Design review of the part built by this model. Coordinates are the model's own, in mm. A direction names the side the tool comes from. Give positions to 0.01 mm unless a question says otherwise; leave off trailing zeros. Loops run counter-clockwise (first coordinate to the right, second up) from the corner with the lowest first, then second, coordinate; pieces in that order, holes last. Notation, with made-up numbers: M 16,22.25 L 61,22.25 A18 cw 61,45.25 Z; hole C 2.5,82.5 d5. An arc over 180 degrees is marked long. Answer as CSV lines item,"result".
```python
from build123d import *

# Parameters (mm, degrees)
BOSS_EXTRUDE1_DEPTH = 36
SKETCH2_W           = 16.184746641
SKETCH2_H           = 32
CUT_EXTRUDE1_DEPTH  = 36
CUT_EXTRUDE2_DEPTH  = 36
SKETCH4_3_R         = 12
CUT_EXTRUDE3_DEPTH  = 36
BOSS_EXTRUDE2_START = 14
SKETCH4_4_R         = 18
SKETCH4_4_R_2       = 12
BOSS_EXTRUDE2_DEPTH = 14
SKETCH5_R           = 4
CUT_EXTRUDE4_DEPTH  = 14
FILLET2_R           = 8
SKETCH9_W           = 12
SKETCH9_H           = 4
BOSS_EXTRUDE3_DEPTH = 12
CUT_EXTRUDE5_DEPTH  = 53


with BuildPart() as part:
    # Sketch1 → Boss-Extrude1 (new body)
    with BuildSketch(Plane(origin=(0, 0, 0), x_dir=(1, 0, 0), z_dir=(0, 1, 0))):
        Polygon((0, 0), (66, 0), (66, 6), (6, 6), (6, 46), (-14, 46), (-14, 14), (0, 14), align=None)
    extrude(amount=BOSS_EXTRUDE1_DEPTH)

    # Sketch2 → Cut-Extrude1 (cut)
    with BuildSketch(Plane(origin=(0, 36, 0), x_dir=(1, 0, 0), z_dir=(0, 1, 0))):
        with Locations((-8.092373321, 30)):
            Rectangle(SKETCH2_W, SKETCH2_H)
    extrude(amount=-CUT_EXTRUDE1_DEPTH, mode=Mode.SUBTRACT)

    # Sketch4 → Cut-Extrude2 (cut)
    with BuildSketch(Plane.ZY):
        with BuildLine():
            ThreePointArc((-23, 0), (-41, 18), (-23, 36))
            Line((-23, 36), (-46, 36))
            Line((-46, 36), (-46, 0))
            Line((-46, 0), (-23, 0))
        make_face()
    extrude(amount=-CUT_EXTRUDE2_DEPTH, mode=Mode.SUBTRACT)

    # Sketch4_3 → Cut-Extrude3 (cut)
    with BuildSketch(Plane.ZY):
        with Locations((-23, 18)):
            Circle(SKETCH4_3_R)
    extrude(amount=-CUT_EXTRUDE3_DEPTH, mode=Mode.SUBTRACT)

    # Sketch4_4 → Boss-Extrude2 (add)
    with BuildSketch(Plane.ZY.offset(BOSS_EXTRUDE2_START)):
        with Locations((-23, 18)):
            Circle(SKETCH4_4_R)
        with Locations((-23, 18)):
            Circle(SKETCH4_4_R_2, mode=Mode.SUBTRACT)
    extrude(amount=-BOSS_EXTRUDE2_DEPTH)

    # Sketch5 → Cut-Extrude4 (cut)
    with BuildSketch(Plane(origin=(0, 0, -6), x_dir=(-1, 0, 0), z_dir=(0, 0, -1))):
        with Locations((-58, 28)):
            Circle(SKETCH5_R)
        with Locations((-58, 8)):
            Circle(SKETCH5_R)
        with BuildLine():
            Line((-43, 22), (-35, 22))
            ThreePointArc((-35, 22), (-31, 18), (-35, 14))
            Line((-35, 14), (-43, 14))
            ThreePointArc((-43, 14), (-47, 18), (-43, 22))
        make_face()
    extrude(amount=-CUT_EXTRUDE4_DEPTH, mode=Mode.SUBTRACT)

    # Fillet2
    fillet2_edges = [part.edges().sort_by_distance(p)[0] for p in [
        (66, 0, -3),
        (66, 36, -3),
    ]]
    fillet(fillet2_edges, radius=FILLET2_R)

    # Sketch9 → Boss-Extrude3 (add)
    with BuildSketch(Plane(origin=(0, 0, -6), x_dir=(-1, 0, 0), z_dir=(0, 0, -1))):
        with Locations((-12, 31)):
            Rectangle(SKETCH9_W, SKETCH9_H)
        with Locations((-12, 5)):
            Rectangle(SKETCH9_W, SKETCH9_H)
    extrude(amount=BOSS_EXTRUDE3_DEPTH)

    # Sketch10 → Cut-Extrude5 (cut)
    with BuildSketch(Plane.XZ.offset(-3)):
        Polygon((18, -6), (6, -18), (14.583968048, -28.688637826), (24.603794653, -16.204919433), align=None)
    extrude(amount=-CUT_EXTRUDE5_DEPTH, mode=Mode.SUBTRACT)


solid = part.part
```
1. The part is to be moulded in two halves that separate along Y. For faces 5 (the flat face through (66, 18, -3)), 6 (the cylindrical face through (31, 18, -3)), 7 (the flat face through (9, 33, -9)), say which applies: pulls with the +Y half, pulls with the -Y half, needs draft (parallel to the pull), parting line crosses it, or undercut.
Answer block:
face 5,"needs draft"
face 6,"undercut"
face 7,"pulls with the +Y half"
2. We need section A-A, the plane y = 18. Write out the cut boundary in (x, z), plus the area to 3 significant figures.
Answer block:
outline,"M -14,-41 L 6,-41 L 6,-35 L -14,-35 Z; M -14,-11 L 6,-11 L 6,-6 L 31,-6 L 31,0 L 0,0 L 0,-5 L -14,-5 Z; M 47,-6 L 66,-6 L 66,0 L 47,0 Z"
area,"534 mm²"
3. We need section C-C, the plane z = -19. Write out the cut boundary in (x, y).
Answer block:
outline,"M -14,0.45 L 0,0.45 L 0,0 L 6,0 L 6,6.69 L -14,6.69 Z; M -14,29.31 L 6,29.31 L 6,36 L 0,36 L 0,35.55 L -14,35.55 Z"
4. For P1, Ø5, axis at y = 30, z = -9, coming from the +X side; P2, Ø3.5, axis at x = 10, z = -14.5, coming from the -Y side; P3, Ø1, axis at y = 6, z = -20.5, coming from the +X side, all flat-tipped, find the tip position at first contact; note any pin that passes through.
Answer block:
P1,"x = 17.5"
P2,"y = 3"
P3,"x = 6"
5. We need section D-D, the plane z = -24. Write out the cut boundary in (x, y).
Answer block:
outline,"M -14,0.03 L 6,0.03 L 6,6.04 L -14,6.04 Z; M -14,29.96 L 6,29.96 L 6,35.97 L -14,35.97 Z"
6. We need section B-B, the plane x = 38. Write out the cut boundary in (y, z), plus the area to 3 significant figures.
Answer block:
outline,"M 0,-6 L 14,-6 L 14,0 L 0,0 Z; M 22,-6 L 36,-6 L 36,0 L 22,0 Z"
area,"168 mm²"
7. To check wall thickness, follow L1, parallel to Y at x = 58, z = -3.3; L2, parallel to Y at x = -9, z = -23.5; L3, parallel to Z at x = 26, y = 21.5. State the ranges of each line that lie inside material, in increasing order. Write a range as [from, to].
Answer block:
L1,"[0, 4], [12, 24], [32, 36]"
L2,"[0.01, 6.01], [29.99, 35.99]"
L3,"[-6, 0]"
8. For faces 1 (the flat face through (39, 14, -3)), 2 (the flat face through (9, 3, -9)), 3 (the flat face through (0, 18, -4)), 4 (the flat face through (6, 13.7, -11.6)), list the 3-axis set-ups (+Z, -Z, +X, -X, +Y, -Y) from which the entire face can be reached by the end or side of a thin tool; tool diameter is ignored.
Answer block:
face 1,"+Z, -Z"
face 2,"-Z, +X, -Y"
face 3,"+Z, -X"
face 4,"-Z, +X"
